```python
from build123d import *

# Parameters (mm, degrees)
EXTRUDE_1_DEPTH        = 94
EXTRUDE_2_DEPTH        = 94
SKETCH_4_R             = 1.5
CUT_EXTRUDE_1_DEPTH    = 128.125921826
CUT_EXTRUDE_START      = -3
SKETCH_5_R             = 3
CUT_EXTRUDE_2_DEPTH    = 131.125921826
SKETCH_6_W             = 21.2
SKETCH_6_H             = 5.25
CUT_EXTRUDE_3_DEPTH    = 2.76
PATTERN_LINEAR_1_COUNT = 9
PATTERN_LINEAR_1_PITCH = 10
FILLET_2_R             = 2


with BuildPart() as part:
    # 草图3 → 凸台-拉伸1 (new body)
    with BuildSketch(Plane.XY):
        with BuildLine():
            Line((0, 0), (-75, 0))
            ThreePointArc((-75, 0), (-82.071067812, -2.928932188), (-85, -10))
            Line((-85, -10), (-75, -10))
            Line((-75, -10), (0, -10))
            Line((0, -10), (0, 0))
        make_face()
        with BuildLine():
            Line((75, 0), (0, 0))
            Line((0, 0), (0, -10))
            Line((0, -10), (75, -10))
            Line((75, -10), (85, -10))
            ThreePointArc((85, -10), (82.071067812, -2.928932188), (75, 0))
        make_face()
    extrude(amount=EXTRUDE_1_DEPTH)

    # 草图2 → 凸台-拉伸2 (add, through all)
    with BuildSketch(Plane.XY):
        Polygon((7.84, 9.32), (10.6, 6.56), (7.84, 3.8), (7.84, 0), (-7.84, 0), (-7.84, 3.8), (-10.6, 6.56), (-7.84, 9.32), align=None)
    extrude(amount=EXTRUDE_2_DEPTH)

    # 草图4 → 切除-拉伸1 (cut, through all)
    with BuildSketch(Plane(origin=(0, 0, 0), x_dir=(1, 0, 0), z_dir=(0, 1, 0))):
        with Locations(Location((-65, -12, 0), (0, 0, 180))):
            Circle(SKETCH_4_R)
        with Locations(Location((-10, -12, 0), (0, 0, 180))):
            Circle(SKETCH_4_R)
        with Locations((10, -12)):
            Circle(SKETCH_4_R)
        with Locations((65, -12)):
            Circle(SKETCH_4_R)
        with Locations(Location((65, -82, 0), (0, 0, 180))):
            Circle(SKETCH_4_R)
        with Locations(Location((10, -82, 0), (0, 0, 180))):
            Circle(SKETCH_4_R)
        with Locations((-65, -82)):
            Circle(SKETCH_4_R)
        with Locations((-10, -82)):
            Circle(SKETCH_4_R)
    extrude(amount=-CUT_EXTRUDE_1_DEPTH, mode=Mode.SUBTRACT)

    # 草图5 → 切除-拉伸2 (cut, through all)
    with BuildSketch(Plane(origin=(0, 0, 0), x_dir=(1, 0, 0), z_dir=(0, 1, 0)).offset(CUT_EXTRUDE_START)):
        with Locations(Location((-65, -12, 0), (0, 0, 180))):
            Circle(SKETCH_5_R)
        with Locations(Location((-10, -12, 0), (0, 0, 43.945519562))):
            Circle(SKETCH_5_R)
        with Locations((10, -12)):
            Circle(SKETCH_5_R)
        with Locations((65, -12)):
            Circle(SKETCH_5_R)
        with Locations(Location((65, -82, 0), (0, 0, 180))):
            Circle(SKETCH_5_R)
        with Locations(Location((10, -82, 0), (0, 0, 281.536959033))):
            Circle(SKETCH_5_R)
        with Locations((-10, -82)):
            Circle(SKETCH_5_R)
        with Locations((-65, -82)):
            Circle(SKETCH_5_R)
    extrude(amount=CUT_EXTRUDE_2_DEPTH, mode=Mode.SUBTRACT)

    # 草图6 → 切除-拉伸3 (cut)
    with BuildSketch(Plane(origin=(0, 9.32, 0), x_dir=(1, 0, 0), z_dir=(0, 1, 0))):
        with Locations((0, -7.375)):
            Rectangle(SKETCH_6_W, SKETCH_6_H)
    cut_extrude_3 = extrude(amount=-CUT_EXTRUDE_3_DEPTH, mode=Mode.SUBTRACT)

    # 阵列(线性)1: 切除-拉伸3 ×9
    with Locations(*[(0, 0, i * PATTERN_LINEAR_1_PITCH) for i in range(1, PATTERN_LINEAR_1_COUNT)]):
        add(cut_extrude_3, mode=Mode.SUBTRACT)

    # 圆角2
    fillet_2_edges = [part.edges().sort_by_distance(p)[0] for p in [
        (-9.22, 7.94, 0),
        (-9.22, 5.18, 0),
        (-7.84, 1.9, 0),
        (7.84, 1.9, 0),
        (9.22, 5.18, 0),
        (9.22, 7.94, 0),
        (-9.22, 7.94, 94),
        (-9.22, 5.18, 94),
        (-7.84, 1.9, 94),
        (7.84, 1.9, 94),
        (9.22, 5.18, 94),
        (9.22, 7.94, 94),
    ]]
    fillet(fillet_2_edges, radius=FILLET_2_R)


solid = part.part
```
CAD build for the part. Positions are in the model's coordinates, mm. A direction names the side the tool comes from. Give positions to 0.01 mm unless a question says otherwise; leave off trailing zeros. Order: outer loops, then holes, each group sorted by start corner. A loop starts at its lowest first (then second) coordinate and runs counter-clockwise, first axis right, second up.
(1) Mould opens along Z. For faces 1 (the cylindrical face through (-8.5, -6.45, 12.07)), 2 (the flat face through (-1, -10, 46)) say: released by +Z, released by -Z, zero draft, split by the parting line, or undercut.
(2) Saw through at C-C, the plane x = -15. Give the cut face in (y, z), then the cut area to 3 significant figures.
(3) Flat gauge pins, fed straight in: pin 1 (1.1 mm diameter, centred on y = 2.5, z = 45.5, fed in from -X); pin 2 (8 mm diameter, centred on y = -3, z = 12.5, fed in from +X); pin 3 (3 mm diameter, centred on x = 64, z = 82, fed in from +Y); pin 4 (2.5 mm diameter, centred on x = -65, z = 82, fed in from +Y). Where does each tip first touch, or does it go through?
(4) Drill centre lines: L1, parallel to Z at x = -65, y = -2.2; L2, parallel to Z at x = 65, y = -5; L3, parallel to X at y = -8.5, z = 82. Where is each one in solid material? Low to high.
(5) Saw through at A-A, the plane z = 62. Give the cut face in (x, y), then the cut area to 3 significant figures.
(6) Saw through at D-D, the plane z = 87. Give the cut face in (x, y), then the cut area to 3 significant figures.
(7) Tool access for faces 3 (the flat face through (7.84, 2, 47)), 4 (the cylindrical face through (82.15, -3.01, 46.34)), 5 (the flat face through (-7.84, 2, 88)), 6 (the cylindrical face through (-67.4, -1.5, 83.8)), 7 (the flat face through (0, 6.56, 67)): list every direction of +Z, -Z, +X, -X, +Y, -Y with a clear straight run to the whole face (end or side of a thin tool).
(8) Saw through at B-B, the plane y = 1.75. Give the cut face in (x, z).
Results found:
1. face 1: undercut
1. face 2: zero draft
2. outline: (-10, 0) - (0, 0) - (0, 94) - (-10, 94) - close
2. area: 940 mm2
3. pin 1: stops at x = -7.84
3. pin 2: stops at x = 84.54
3. pin 3: stops at y = -3
3. pin 4: passes through
4. L1: z = 0 to 9, 15 to 79, 85 to 94
4. L2: z = 0 to 10.5, 13.5 to 80.5, 83.5 to 94
4. L3: x = -84.89 to -66.5, -63.5 to -11.5, -8.5 to 8.5, 11.5 to 63.5, 66.5 to 84.89
5. outline: (-85, -10) - (85, -10) arc R10 ccw to (75, 0) - (7.84, 0) - (7.84, 3.8) - (10.6, 6.56) - (7.84, 9.32) - (-7.84, 9.32) - (-10.6, 6.56) - (-7.84, 3.8) - (-7.84, 0) - (-75, 0) arc R10 ccw to start
5. area: 1,820 mm2
6. outline: (-85, -10) - (85, -10) arc R10 ccw to (75, 0) - (7.84, 0) - (7.84, 3.8) - (10.6, 6.56) - (-10.6, 6.56) - (-7.84, 3.8) - (-7.84, 0) - (-75, 0) arc R10 ccw to start
6. area: 1,770 mm2
7. face 3: +Z, -Z, +X
7. face 4: +Z, -Z, +X, +Y
7. face 5: +Z, -Z, -X
7. face 6: +Y
7. face 7: +X, -X, +Y
8. outline: (-7.84, 2) arc R2 ccw to (-5.84, 0) - (5.84, 0) arc R2 ccw to (7.84, 2) - (7.84, 9.92) arc R3 cw to (7.84, 14.08) - (7.84, 79.92) arc R3 cw to (7.84, 84.08) - (7.84, 92) arc R2 ccw to (5.84, 94) - (-5.84, 94) arc R2 ccw to (-7.84, 92) - (-7.84, 84.08) arc R3 cw to (-7.84, 79.92) - (-7.84, 14.08) arc R3 cw to (-7.84, 9.92) - close
